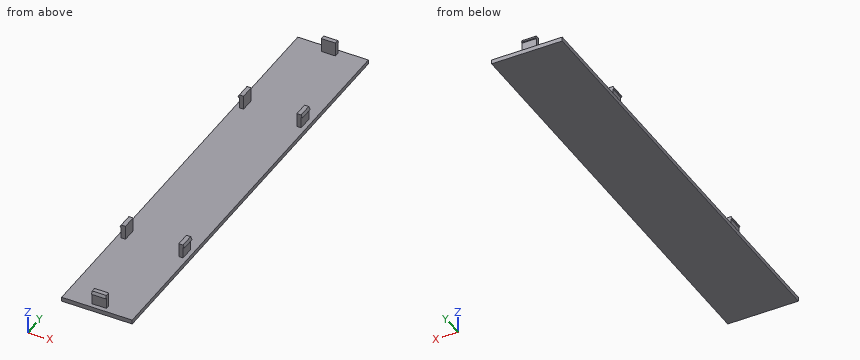
```python
from build123d import *

# Parameters (mm, degrees)
SKETCH2_W            = 154.25
SKETCH2_H            = 25
BOSS_EXTRUDE1_DEPTH  = 1.5
SKETCH3_W            = 5
SKETCH3_H            = 1.5
BOSS_EXTRUDE2_DEPTH  = 5
BOSS_EXTRUDE3_DEPTH  = 5
SKETCH5_W            = 1.5
SKETCH5_H            = 5
BOSS_EXTRUDE4_DEPTH  = 5
BOSS_EXTRUDE5_DEPTH  = 5
MIRROR5_COPY_1_DEPTH = 5


with BuildPart() as part:
    # Sketch2 → Boss-Extrude1 (new body)
    with BuildSketch(Plane(origin=(0, 0, 0), x_dir=(0, 1, 0), z_dir=(0, 0, 1))):
        with Locations((77.125, 12.5)):
            Rectangle(SKETCH2_W, SKETCH2_H)
    extrude(amount=BOSS_EXTRUDE1_DEPTH)

    # Sketch3 → Boss-Extrude2 (add)
    with BuildSketch(Plane.XY.offset(1.5)):
        with Locations((-12.5, 2.3)):
            Rectangle(SKETCH3_W, SKETCH3_H)
    boss_extrude2 = extrude(amount=BOSS_EXTRUDE2_DEPTH)

    # Sketch4 → Boss-Extrude3 (add)
    with BuildSketch(Plane.YZ.offset(-10)):
        Polygon((1.55, 6.5), (1.05, 5.5), (1.55, 5.5), align=None)
    boss_extrude3 = extrude(amount=-BOSS_EXTRUDE3_DEPTH)

    # Sketch5 → Boss-Extrude4 (add)
    with BuildSketch(Plane.XY.offset(1.5)):
        with Locations((-2.3, 38.5625)):
            Rectangle(SKETCH5_W, SKETCH5_H)
        with Locations((-2.3, 115.6875)):
            Rectangle(SKETCH5_W, SKETCH5_H)
    boss_extrude4 = extrude(amount=BOSS_EXTRUDE4_DEPTH)

    # Sketch6 → Boss-Extrude5 (add)
    with BuildSketch(Plane.XZ.offset(-36.0625)):
        Polygon((-1.55, 6.5), (-1.05, 5.5), (-1.55, 5.5), align=None)
    boss_extrude5 = extrude(amount=-BOSS_EXTRUDE5_DEPTH)

    # Mirror2: Boss-Extrude5 across plane
    add(boss_extrude5.mirror(Plane(origin=(0, 77.125, 0), x_dir=(0, 0, 1), z_dir=(0, -1, 0))))

    # Mirror3: Boss-Extrude2 across plane
    add(boss_extrude2.mirror(Plane(origin=(0, 77.125, 0), x_dir=(0, 0, 1), z_dir=(0, -1, 0))))

    # Mirror4: Boss-Extrude3 across plane
    add(boss_extrude3.mirror(Plane(origin=(0, 77.125, 0), x_dir=(0, 0, 1), z_dir=(0, -1, 0))))

    # Mirror5: Boss-Extrude4, Boss-Extrude5 across plane
    add(boss_extrude4.mirror(Plane(origin=(-12.5, 0, 0), x_dir=(0, 0, 1), z_dir=(1, 0, 0))))
    add(boss_extrude5.mirror(Plane(origin=(-12.5, 0, 0), x_dir=(0, 0, 1), z_dir=(1, 0, 0))))

    # Mirror5 copy 1 sketch → Mirror5 copy 1 (add)
    with BuildSketch(Plane(origin=(-25, 118.1875, 0), x_dir=(-1, 0, 0), z_dir=(0, 1, 0))):
        Polygon((-1.55, 6.5), (-1.05, 5.5), (-1.55, 5.5), align=None)
    extrude(amount=-MIRROR5_COPY_1_DEPTH)


solid = part.part
```
Here's how the part is built. I have some questions about the finished solid (model axes, mm). Give positions to 0.01 mm unless a question says otherwise; leave off trailing zeros. Order: outer loops, then holes, each group sorted by start corner. A loop starts at its lowest first (then second) coordinate and runs counter-clockwise, first axis right, second up. Notation, with made-up numbers: M 55,22.5 L 112,22.5 A31 ccw 112,47.5 Z; hole C 15.25,18.25 d9. An arc over 180 degrees is marked long. Use a Markdown table: item, result. Add a question column.
1. Suppose I cut it at B-B (y = 116.5). List the corners of the cut face in (x, z) for me, and give its area (3 significant figures).
2. Suppose I cut it at A-A (z = 4). List the corners of the cut face in (x, y) for me, and give its area (3 significant figures).
3. I need wall thicknesses on probe 1 along Y at (x, z) = (-10.5, 2); probe 2 along Z at (x, y) = (-14.75, 21). Which ranges of each line are inside material? Lowest first, please. Write a range as from..to.
4. Suppose I cut it at C-C (x = -13.25). List the corners of the cut face in (y, z) for me, and give its area (3 significant figures).
5. For pin 1 Ø3 at (x, z) = (-13.5, 4.5) entering from +Y; pin 2 Ø1.6 at (x, z) = (-2, 4.5) entering from -Y; pin 3 Ø2 at (y, z) = (38.5, 3.5) entering from -X, each with a flat end and sliding along its axis, tell me the tip position at first contact or that it passes through.
6. Suppose I cut it at D-D (x = -6). List the corners of the cut face in (y, z) for me.
Results list:
| question | item | result |
|---|---|---|
| 1 | outline | M -25,0 L 0,0 L 0,1.5 L -1.55,1.5 L -1.55,5.5 L -1.05,5.5 L -1.55,6.5 L -3.05,6.5 L -3.05,1.5 L -21.95,1.5 L -21.95,6.5 L -23.45,6.5 L -23.95,5.5 L -23.45,5.5 L -23.45,1.5 L -25,1.5 Z |
| 1 | area | 53.0 mm² |
| 2 | outline | M -23.45,36.06 L -21.95,36.06 L -21.95,41.06 L -23.45,41.06 Z; M -23.45,113.19 L -21.95,113.19 L -21.95,118.19 L -23.45,118.19 Z; M -15,1.55 L -10,1.55 L -10,3.05 L -15,3.05 Z; M -15,151.2 L -10,151.2 L -10,152.7 L -15,152.7 Z; M -3.05,36.06 L -1.55,36.06 L -1.55,41.06 L -3.05,41.06 Z; M -3.05,113.19 L -1.55,113.19 L -1.55,118.19 L -3.05,118.19 Z |
| 2 | area | 45.0 mm² |
| 3 | probe 1 | y = 1.55..3.05, 151.2..152.7 |
| 3 | probe 2 | z = 0..1.5 |
| 4 | outline | M 0,0 L 154.25,0 L 154.25,1.5 L 152.7,1.5 L 152.7,5.5 L 153.2,5.5 L 152.7,6.5 L 151.2,6.5 L 151.2,1.5 L 3.05,1.5 L 3.05,6.5 L 1.55,6.5 L 1.05,5.5 L 1.55,5.5 L 1.55,1.5 L 0,1.5 Z |
| 4 | area | 247 mm² |
| 5 | pin 1 | stops at y = 153.2 |
| 5 | pin 2 | stops at y = 36.06 |
| 5 | pin 3 | stops at x = -23.45 |
| 6 | outline | M 0,0 L 154.25,0 L 154.25,1.5 L 0,1.5 Z |
